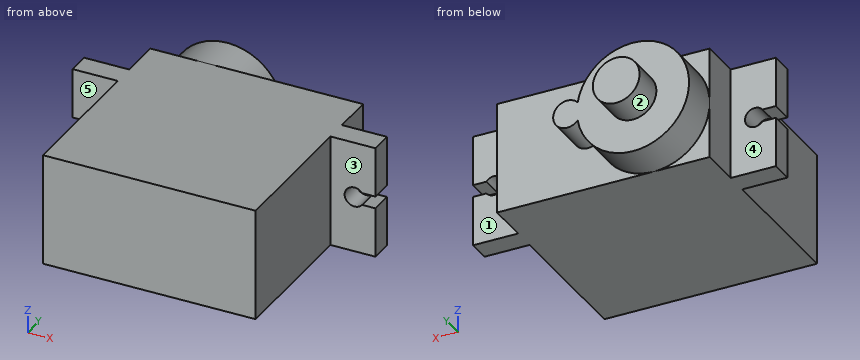
Autodesk Inventor part; units mm, degrees
ref_plane "YZ Plane" through (0, 0, 0) normal (1, 0, 0) x (0, 1, 0)
ref_plane "XZ Plane" through (0, 0, 0) normal (0, 1, 0) x (-1, 0, 0)
ref_plane "XY Plane" through (0, 0, 0) normal (0, 0, 1) x (1, 0, 0)
sketch "Sketch1" plane through (0, 0, 0) normal (0, 0, 1) x (1, 0, 0)
  line L0 (0, 0) -> (-11.375, 0)
  line L1 (-11.375, 0) -> (-11.375, 15.6)
  line L2 (-11.375, 15.6) -> (-16.2, 15.6)
  line L3 (-16.2, 15.6) -> (-16.2, 18)
  line L4 (-16.2, 18) -> (-11.375, 18)
  line L5 (-11.375, 18) -> (-11.375, 22.4)
  line L6 (-11.375, 22.4) -> (11.375, 22.4)
  line L7 (11.375, 22.4) -> (11.375, 18)
  line L8 (11.375, 18) -> (16.2, 18)
  line L9 (16.2, 18) -> (16.2, 15.6)
  line L10 (16.2, 15.6) -> (11.375, 15.6)
  line L11 (11.375, 15.6) -> (11.375, 0)
  line L12 (11.375, 0) -> (0, 0)
  dimension "d0" = 11.375
  dimension "d1" = 15.6
  dimension "d2" = 4.825
  dimension "d3" = 2.4
  dimension "d4" = 4.4
  dimension "d5" = 22.75
  dimension "d7" = 4.825
  dimension "d8" = 2.4
  dimension "d9" = 18
extrude "Extrusion1" add sketch "Sketch1" along normal blind 12
sketch "Sketch2" plane through (-11.375, 22.4, 0) normal (0, 1, 0) x (1, 0, 0)
  line L0 (0, -12) -> (22.75, -12)
  line L1 (0, 0) -> (22.75, 0)
  line L2 (0, 0) -> (0, -12)
  arc A0 (11.9166, -5.003) -> (11.9166, -6.997) centre (6, -6) ccw
  arc A1 (11.9166, -6.997) -> (11.9166, -5.003) centre (13.0373, -6) ccw
  point P0 (11.375, 0)
  dimension "d13" = 3
extrude "Extrusion2" add sketch "Sketch2" along normal blind 4.3 contours A0 A1
sketch "Sketch3" plane through (-11.375, 26.7, 0) normal (0, 1, 0) x (1, 0, 0)
  arc A0 (11.9166, -5.003) -> (11.9166, -6.997) centre (6, -6) ccw
  circle A1 centre (6, -6) radius 2.5
  point P0 (11.375, 0)
  dimension "d16" = 5
extrude "Extrusion3" add sketch "Sketch3" along normal blind 3.5
sketch "Sketch4" plane through (-16.2, 18, 0) normal (0, 1, 0) x (1, 0, 0)
  line L0 (0, 0) -> (0, -12)
  line L1 (27.575, -12) -> (32.4, -12)
  line L2 (32.4, 0) -> (32.4, -12)
  line L3 (27.575, 0) -> (32.4, 0)
  line L4 (27.575, 0) -> (27.575, -12)
  arc A0 (1.4254, -6.65) -> (1.4254, -5.35) centre (2.25, -6) ccw
  arc A1 (30.9746, -5.35) -> (30.9746, -6.65) centre (30.15, -6) ccw
  line L5 (0, 0) -> (0, -12) construction
  line L6 (0, -6) -> (32.4, -6) construction
  line L7 (32.4, 0) -> (32.4, -12) construction
  line L8 (0, -5.35) -> (1.4254, -5.35)
  line L9 (0, -6.65) -> (1.4254, -6.65)
  line L10 (32.4, -5.35) -> (30.9746, -5.35)
  line L11 (32.4, -6.65) -> (30.9746, -6.65)
  line L12 (0, -5.35) -> (-0.3532, -5.35)
  line L13 (-0.3532, -5.35) -> (-0.3532, -6.65)
  line L14 (-0.3532, -6.65) -> (0, -6.65)
  line L15 (32.4, -5.35) -> (32.7834, -5.35)
  line L16 (32.7834, -5.35) -> (32.7834, -6.65)
  line L17 (32.7834, -6.65) -> (32.4, -6.65)
  point P0 (16.2, 0)
  dimension "d19" = 2.1
  dimension "d20" = 2.1
  dimension "d21" = 27.9
  dimension "d22" = 2.25
  dimension "d23" = 1.3
  dimension "d25" = 0.65
  dimension "d26" = 1.3
  dimension "d27" = 0.65
extrude "Extrusion4" cut sketch "Sketch4" against normal up to next contours L8 A0 L9 L0 | L0 L14 L13 L12 | L11 A1 L10 L2 | L2 L15 L16 L17
properties part number "MicroServo_Motor"
For this review, take the finished solid that the model builds, in its own axes (mm). Face numbers are marked on the shaded views. A direction names the side the tool comes from. Round coordinates to 2 decimals unless told otherwise and drop trailing zeros. Order: outer loops, then holes, each group sorted by start corner. A loop starts at its lowest first (then second) coordinate and runs counter-clockwise, first axis right, second up. Notation, with made-up numbers: M 31.25,16.25 L 84.25,16.25 A23 ccw 84.25,52.25 Z; hole C -23.5,35 d4. An arc over 180 degrees is marked long. Write each question's results on one line, items separated by ' | '. Start each with the question number.
1. Add section D-D (x = -2). State the section outline as (y, z) points, then the cut area to 3 significant figures.
2. Clearance check with flat-ended pins moving along their axes: pin 1 Ø5 at (y, z) = (23, 8.5) entering from -X (3 decimals); pin 2 Ø5.5 at (x, z) = (-14, 4) entering from +Y; pin 3 Ø1 at (x, y) = (7.5, 23.5) entering from -Z; pin 4 Ø1.4 at (x, z) = (13.5, 3.5) entering from -Y. State where each tip first meets the part, or that it passes through.
3. Tool access review of the marked faces 1, 2, 3, 4 and 5: name each direction out of +Z, -Z, +X, -X, +Y, -Y from which nothing blocks a thin tool from reaching the whole face with its end or side.
4. Add section C-C (y = 7.5). State the section outline as (x, z) points (3 decimals).
5. Add section A-A (x = -13.95). State the section outline as (y, z) points.
6. To check wall thickness, follow L1, parallel to Z at x = 13.95, y = 16.8; L2, parallel to Y at x = 6, z = 10; L3, parallel to X at y = 3, z = 1.5 (3 decimals). State the ranges of each line that lie inside material, in increasing order. Write a range as [from, to].
7. Add section B-B (z = 1). State the section outline as (x, y) points (3 decimals), then the cut area to 3 significant figures.
Output values:
1) outline: M 0,0 L 22.4,0 L 22.4,1.04 L 26.7,1.04 L 26.7,10.96 L 22.4,10.96 L 22.4,12 L 0,12 Z | area: 311 mm^2
2) pin 1: x = -11.375 | pin 2: y = 22.4 | pin 3: through | pin 4: y = 15.6
3) face 1: +Z, -Z, +X, +Y | face 2: +Y | face 3: +Z, -Z, +X, -Y | face 4: +Z, -Z, -X, +Y | face 5: +Z, -Z, -X, -Y
4) outline: M -11.375,0 L 11.375,0 L 11.375,12 L -11.375,12 Z
5) outline: M 15.6,0 L 18,0 L 18,4.95 L 15.6,4.95 Z; M 15.6,7.05 L 18,7.05 L 18,12 L 15.6,12 Z
6) L1: [0, 4.95], [7.05, 12] | L2: [0, 22.4] | L3: [-11.375, 11.375]
7) outline: M -16.2,15.6 L -11.375,15.6 L -11.375,0 L 11.375,0 L 11.375,15.6 L 16.2,15.6 L 16.2,18 L 11.375,18 L 11.375,22.4 L -2.058,22.4 L -2.058,26.7 L -8.692,26.7 L -8.692,22.4 L -11.375,22.4 L -11.375,18 L -16.2,18 Z | area: 561 mm^2
